Autodesk Inventor part; units mm, degrees
ref_plane "YZ Plane" through (0, 0, 0) normal (1, 0, 0) x (0, 1, 0)
ref_plane "XZ Plane" through (0, 0, 0) normal (0, 1, 0) x (-1, 0, 0)
ref_plane "XY Plane" through (0, 0, 0) normal (0, 0, 1) x (1, 0, 0)
sketch "Sketch2" plane through (0, 0, 0) normal (0, 0, 1) x (1, 0, 0)
  line L0 (-20, 6) -> (20, 6)
  line L1 (20, 6) -> (20, -6)
  line L2 (20, -6) -> (-20, -6)
  line L3 (-20, -6) -> (-20, 6)
  line L4 (-20, 6) -> (20, -6) construction
  line L5 (20, 6) -> (-20, -6) construction
  point P0 (0, 0)
  dimension "d0" = 40
  dimension "d1" = 12
extrude "Extrusion1" add sketch "Sketch2" against normal blind 4
sketch "Sketch3" plane through (0, 0, 0) normal (0, 0, 1) x (1, 0, 0)
  line L0 (0, 0) -> (16.1, 0) construction
  line L1 (0, 0) -> (16.1, 0) construction
  arc A0 (14, -2.1) -> (14, 2.1) centre (14, 0) ccw
  line L2 (2.3812, 0) -> (2.3812, 2.7) construction
  line L3 (2.3812, 2.7) -> (14, 2.1)
  line L4 (2.3812, -2.7) -> (14, -2.1)
  line L5 (0, 0) -> (0, 3.6) construction
  arc A1 (-14, 2.1) -> (-14, -2.1) centre (-14, 0) ccw
  line L6 (-2.3812, 2.7) -> (-14, 2.1)
  line L7 (-2.3812, -2.7) -> (-14, -2.1)
  arc A2 (2.3812, 2.7) -> (-2.3812, 2.7) centre (0, 0) ccw
  arc A3 (-2.3812, -2.7) -> (2.3812, -2.7) centre (0, 0) ccw
  dimension "d10" = 16.1
  dimension "d12" = 2.7
extrude "Extrusion3" cut sketch "Sketch3" against normal blind 2
properties part number "micro_horn_test"
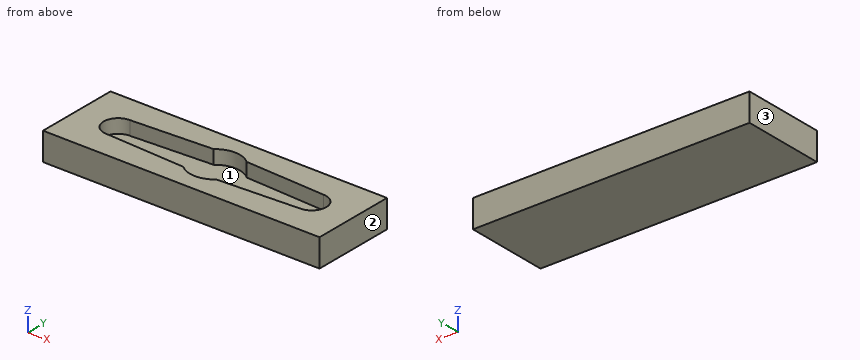
Read the model definition and answer for the solid it produces. Units are mm, in the model's axes. Face numbers are marked on the shaded views. Give positions to 0.01 mm unless a question says otherwise; leave off trailing zeros. Write each loop counter-clockwise with the first axis right and the second up, starting at its lowest first coordinate (ties: lowest second). Pieces come first, ordered by that corner, then holes. Notation, with made-up numbers: (70, 5.5) -> (97, 5.5) arc R33 cw to (97, 38.5) -> close; hole circle Ø8 at (-15, -7.75). An arc over 180 degrees is marked (long way). Answer as a JSON object with one key per item and string values. Group by question number.
1) Find section A-A (z = -1.65). Write down the section's boundary in (x, y).
2) This flat-tipped pin is pushed along its axis until it touches: P1, Ø2, axis at x = -5.5, y = 0.5, coming from the +Z side. Where does it stop, or does it pass through?
3) The mould has two halves that part along X. Classify the marked faces 1, 2 and 3: +X half, -X half, draft (parallel to the pull), parting line (faces both ways), or undercut.
4) Find section B-B (x = -4). Write down the section's boundary in (y, z).
5) Consider L1, parallel to Y at x = 8.5, z = -0.8; L2, parallel to Z at x = 2, y = 0.5; L3, parallel to Y at x = -6, z = -1.8. Determine where each line is inside the solid, lowest interval first. Write a range as from..to.
6) Find section C-C (y = 0). Write down the section's boundary in (x, z), and give its area (3 significant figures).
Values follow:
{
 "1": {"outline": "(-20, -6) -> (20, -6) -> (20, 6) -> (-20, 6) -> close; hole (-14, -2.1) -> (-2.38, -2.7) arc R3.6 ccw to (2.38, -2.7) -> (14, -2.1) arc R2.1 ccw to (14, 2.1) -> (2.38, 2.7) arc R3.6 ccw to (-2.38, 2.7) -> (-14, 2.1) arc R2.1 ccw to start"},
 "2": {"P1": "stops at z = -2"},
 "3": {"face 1": "undercut", "face 2": "+X half", "face 3": "-X half"},
 "4": {"outline": "(-6, -4) -> (6, -4) -> (6, 0) -> (2.62, 0) -> (2.62, -2) -> (-2.62, -2) -> (-2.62, 0) -> (-6, 0) -> close"},
 "5": {"L1": "y = -6..-2.38, 2.38..6", "L2": "z = -4..-2", "L3": "y = -6..-2.51, 2.51..6"},
 "6": {"outline": "(-20, -4) -> (20, -4) -> (20, 0) -> (16.1, 0) -> (16.1, -2) -> (-16.1, -2) -> (-16.1, 0) -> (-20, 0) -> close", "area": "95.6 mm2"}
}
